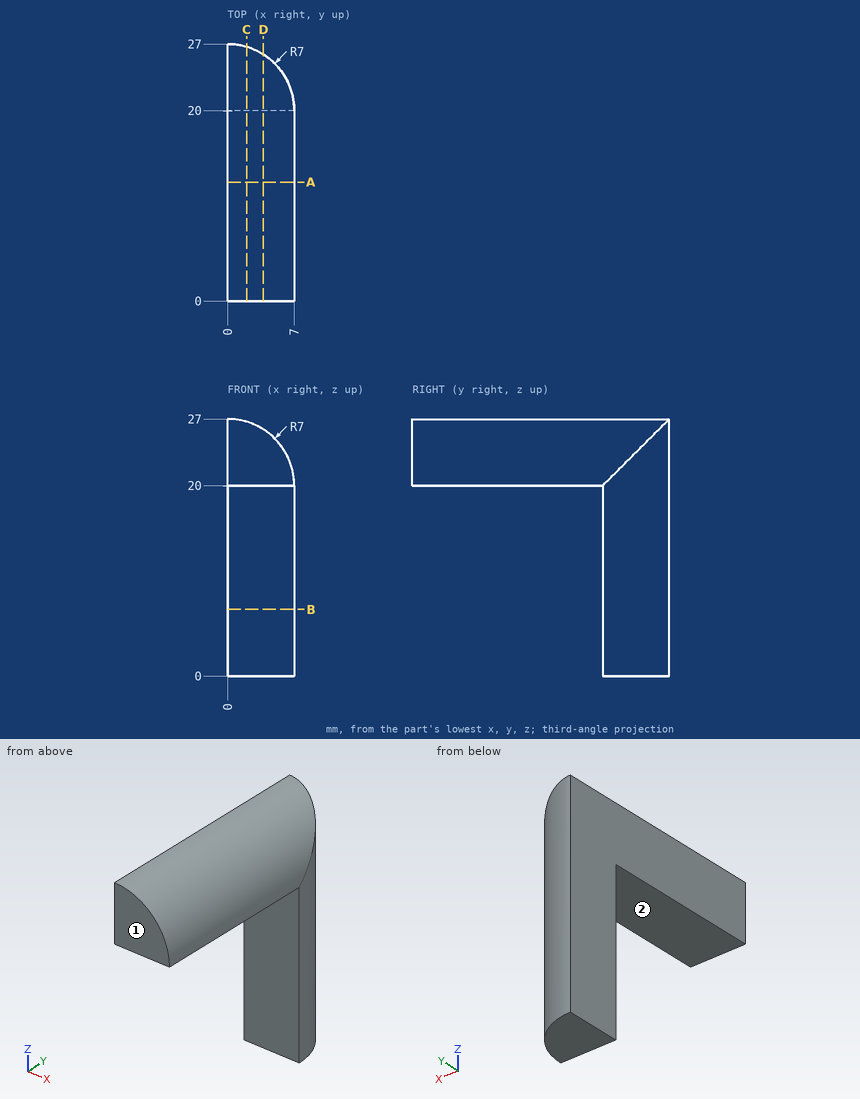
Part print with two shaded views. Sizes in mm from the minimum x, y, z corner. A direction names the side the tool comes from. Round coordinates to 2 decimals unless told otherwise and drop trailing zeros. Loops run counter-clockwise (first coordinate to the right, second up) from the corner with the lowest first, then second, coordinate; pieces in that order, holes last.
Item 1: Pin check, flat tips, straight feed: P1, Ø1, axis at y = 21, z = 20.5, coming from the +X side; P2, Ø1, axis at x = 4, y = 20, coming from the +Z side; P3, Ø1.5, axis at x = 1, z = 15.5, coming from the -Y side; P4, Ø1.5, axis at x = 3, z = 22, coming from the -Y side. Stop position of each tip, or through.
Item 2: Saw through at D-D (x = 3.75). List the corners of the cut face in (y, z).
Item 3: Saw through at C-C (x = 2). List the corners of the cut face in (y, z).
Item 4: Drill centre lines: line 1 along X through (y, z) = (23.5, 9.5); line 2 along Z through (x, y) = (3, 8); line 3 along Y through (x, z) = (3, 25.75). Where is each one in solid material? Low to high.
Item 5: Saw through at A-A (y = 12.5). List the corners of the cut face in (x, z), then the cut area to 3 significant figures.
Item 6: Which spindle directions (+Z, -Z, +X, -X, +Y, -Y) get a long thin tool onto all of the face, cutting with end or side? Do the marked faces 1 and 2. Say none if no direction does.
Worked answers:
1. P1: stops at x = 6.98
1. P2: stops at z = 26.06
1. P3: stops at y = 20
1. P4: stops at y = 0
2. outline: (0, 20) - (20, 20) - (20, 0) - (25.91, 0) - (25.91, 25.91) - (0, 25.91) - close
3. outline: (0, 20) - (20, 20) - (20, 0) - (26.71, 0) - (26.71, 26.71) - (0, 26.71) - close
4. line 1: x = 0 to 6.06
4. line 2: z = 20 to 26.32
4. line 3: y = 0 to 26.32
5. outline: (0, 20) - (7, 20) arc R7 ccw to (0, 27) - close
5. area: 38.5 mm2
6. face 1: +Z, -Z, +X, -X, -Y
6. face 2: -Z, +X, -X, -Y
